```python
from build123d import *

# Parameters (mm, degrees)
SKETCH2_R                       = 11
SKETCH2_R_2                     = 4
BOSS_EXTRUDE1_DEPTH             = 8.8
M2X0_4_TAPPED_HOLE1_D           = 1.6
M2X0_4_TAPPED_HOLE1_DEPTH       = 0.5
BOSS_EXTRUDE3_START             = 14
BOSS_EXTRUDE3_DEPTH             = 5
BOSS_EXTRUDE3_DIRECTION_2_REACH = 39.339


with BuildPart() as part:
    # Sketch1 → Revolve1 (revolve)
    with BuildSketch(Plane.XY, mode=Mode.PRIVATE) as revolve1_sk:
        Polygon((1.5, 4), (1.5, 0), (12.5, 0), (13.8, 4), (13.274256479, 4), (12.136756479, 0.5), (7.1375, 0.5), (6, 4), align=None)
    revolve(revolve1_sk.sketch.rotate(Axis((0, 0, 0), (0, 1, 0)), 90), axis=Axis((0, 0, 0), (0, 1, 0)))

    # Sketch2 → Boss-Extrude1 (add)
    with BuildSketch(Plane(origin=(0, 4, 0), x_dir=(1, 0, 0), z_dir=(0, 1, 0))):
        with Locations(Location((0, 0, 0), (0, 0, 270))):
            Circle(SKETCH2_R)
        with Locations(Location((0, 0, 0), (0, 0, 270))):
            Circle(SKETCH2_R_2, mode=Mode.SUBTRACT)
    extrude(amount=BOSS_EXTRUDE1_DEPTH)

    # M2x0.4 Tapped Hole1
    with Locations(Plane(origin=(0, 0, 0), x_dir=(-1, 0, 0), z_dir=(0, -1, 0))):
        with Locations((0, 8), (0, -8), (-9.25, 0), (9.25, 0)):
            Hole(M2X0_4_TAPPED_HOLE1_D / 2, depth=M2X0_4_TAPPED_HOLE1_DEPTH)

    # Sketch6 → Boss-Extrude3 (add)
    with BuildSketch(Plane(origin=(0, 0, 0), x_dir=(-0.7071067811865477, 0, 0.7071067811865475), z_dir=(-0.7071067811865475, 0, -0.7071067811865477)).offset(BOSS_EXTRUDE3_START)):
        with BuildLine():
            Line((-1.25, 3.475), (1.25, 3.475))
            ThreePointArc((1.25, 3.475), (1.975, 2.75), (1.25, 2.025))
            Line((1.25, 2.025), (-1.25, 2.025))
            ThreePointArc((-1.25, 2.025), (-1.975, 2.75), (-1.25, 3.475))
        make_face()
    extrude(amount=BOSS_EXTRUDE3_DEPTH)

    # Sketch6 → Boss-Extrude3 direction 2 (add, up to next)
    with BuildSketch(Plane(origin=(0, 0, 0), x_dir=(-0.7071067811865477, 0, 0.7071067811865475), z_dir=(-0.7071067811865475, 0, -0.7071067811865477)).offset(BOSS_EXTRUDE3_START), mode=Mode.PRIVATE) as boss_extrude3_direction_2_sk1:
        with BuildLine():
            Line((-1.25, 3.475), (1.25, 3.475))
            ThreePointArc((1.25, 3.475), (1.975, 2.75), (1.25, 2.025))
            Line((1.25, 2.025), (-1.25, 2.025))
            ThreePointArc((-1.25, 2.025), (-1.975, 2.75), (-1.25, 3.475))
        make_face()
    boss_extrude3_direction_2_tool1 = extrude(boss_extrude3_direction_2_sk1.sketch, amount=-BOSS_EXTRUDE3_DIRECTION_2_REACH, mode=Mode.PRIVATE) - part.part
    add(boss_extrude3_direction_2_tool1.solids().sort_by_distance((-9.899495, 2.75, -9.899495))[0])


solid = part.part
```
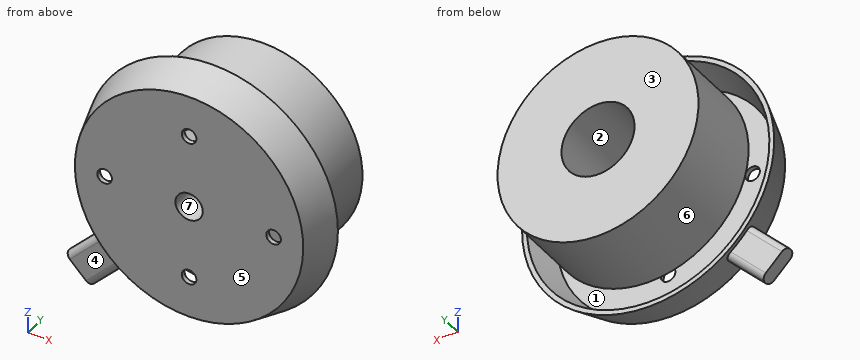
Verification items for the finished model (mm, model axes). Face numbers are marked on the shaded views. A direction names the side the tool comes from. Give positions to 0.01 mm unless a question says otherwise; leave off trailing zeros. Loops run counter-clockwise (first coordinate to the right, second up) from the corner with the lowest first, then second, coordinate; pieces in that order, holes last.
1. Set-up check for the marked faces 1, 2, 3 and 4: record each of +Z, -Z, +X, -X, +Y, -Y from which the full face is reachable in a straight line by a thin tool's end or side.
2. Mould release check, pull along X, two halves, no side actions. Record for the marked faces 5, 6 and 7: released by +X, released by -X, zero draft, split by the parting line, or undercut.
3. Thickness scan on line 1 (Z direction, x = -0.25, y = 6.5); line 2 (Y direction, x = -1, z = 11); line 3 (X direction, y = 0.3, z = -8). Record the ranges inside material, lowest first.
4. Section check C-C, the plane y = 10. Enter the section's corners in (x, z), then the cut area to 3 significant figures.
5. Go/stop test with flat-tipped pins: pin 1 Ø1 at (x, y) = (2.5, 7) entering from -Z; pin 2 Ø4.5 at (x, z) = (-12, -12.5) entering from +Y (3 decimals); pin 3 Ø6.5 at (x, z) = (-11.5, -12) entering from -Y (3 decimals); pin 4 Ø1.8 at (x, z) = (0, 0) entering from -Y. Record where each tip stops, or that it passes through.
6. Section check A-A, the plane x = 0. Count the separate pieces of the cut face and the enclosed holes in it, then the cut area to 3 significant figures.
Geometry says:
1. face 1: none
1. face 2: +Y
1. face 3: +Z, -Z, +X, -X, +Y
1. face 4: -Z, -X, -Y
2. face 5: zero draft
2. face 6: split by the parting line
2. face 7: undercut
3. line 1: z = -11 to -3.99, 3.99 to 11
3. line 2: y = 0 to 0.5
3. line 3: x = -9.73 to -0.8, 0.8 to 9.73
4. outline: circle Ø22 at (0, 0); hole circle Ø8 at (0, 0)
4. area: 330 mm2
5. pin 1: stops at z = -10.82
5. pin 2: stops at y = 3.475
5. pin 3: stops at y = 2.025
5. pin 4: passes through
6. separate pieces: 4
6. enclosed holes: 0
6. area: 172 mm2
